Drawing for the job (mm, zero at the part's lowest x, y, z). Coordinates: 2 decimals unless noted, no trailing zeros. Order: outer loops, then holes, each group sorted by start corner. A loop starts at its lowest first (then second) coordinate and runs counter-clockwise, first axis right, second up.
1) Pin check, flat tips, straight feed: pin 1 Ø5 at (y, z) = (40, 4) entering from +X; pin 2 Ø2.5 at (x, z) = (43, 7.5) entering from -Y; pin 3 Ø3.5 at (x, z) = (12, 8.5) entering from +Y; pin 4 Ø2 at (y, z) = (71, 6) entering from +X. Stop position of each tip, or through.
2) Cut at A-A (y = 43.5). List the corners of the cut face in (x, z), and give its area (3 significant figures).
3) Wall check: L1, parallel to Y at x = 31.5, z = 12.75; L2, parallel to Y at x = 28, z = 13.5; L3, parallel to X at y = 8, z = 13.75. Give the ranges that are in metal, low to high.
4) Cut at C-C (y = 71). List the corners of the cut face in (x, z).
5) Cut at B-B (x = 34). List the corners of the cut face in (y, z).
6) Cut at D-D (z = 1). List the corners of the cut face in (x, y).
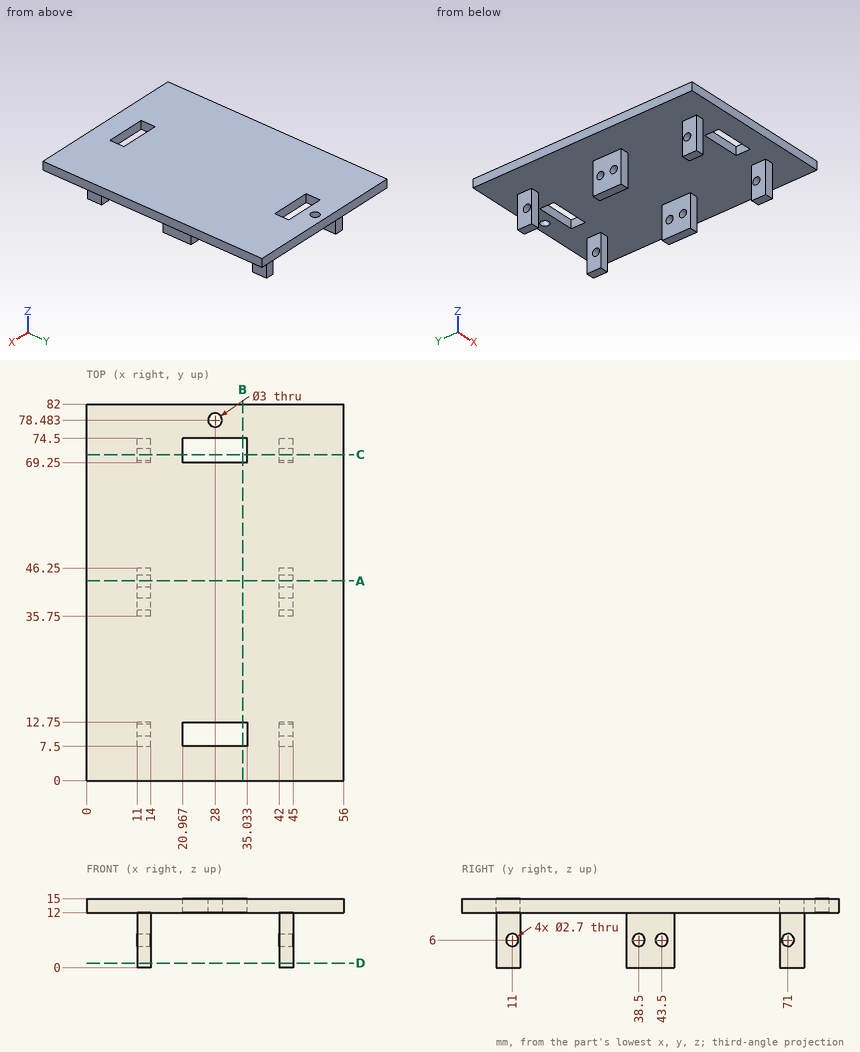
Geometry check:
1. pin 1: stops at x = 45
1. pin 2: stops at y = 7.5
1. pin 3: stops at y = 74.5
1. pin 4: passes through
2. outline: (0, 12) - (11, 12) - (11, 7.35) - (14, 7.35) - (14, 12) - (42, 12) - (42, 7.35) - (45, 7.35) - (45, 12) - (56, 12) - (56, 15) - (0, 15) - close; (11, 0) - (14, 0) - (14, 4.65) - (11, 4.65) - close; (42, 0) - (45, 0) - (45, 4.65) - (42, 4.65) - close
2. area: 224 mm2
3. L1: y = 0 to 7.5, 12.75 to 69.25, 74.5 to 82
3. L2: y = 0 to 7.5, 12.75 to 69.25, 74.5 to 76.98, 79.98 to 82
3. L3: x = 0 to 20.97, 35.03 to 56
4. outline: (0, 12) - (11, 12) - (11, 7.35) - (14, 7.35) - (14, 12) - (20.97, 12) - (20.97, 15) - (0, 15) - close; (11, 0) - (14, 0) - (14, 4.65) - (11, 4.65) - close; (35.03, 12) - (42, 12) - (42, 7.35) - (45, 7.35) - (45, 12) - (56, 12) - (56, 15) - (35.03, 15) - close; (42, 0) - (45, 0) - (45, 4.65) - (42, 4.65) - close
5. outline: (0, 12) - (7.5, 12) - (7.5, 15) - (0, 15) - close; (12.75, 12) - (69.25, 12) - (69.25, 15) - (12.75, 15) - close; (74.5, 12) - (82, 12) - (82, 15) - (74.5, 15) - close
6. outline: (11, 7.5) - (14, 7.5) - (14, 12.75) - (11, 12.75) - close; (11, 35.75) - (14, 35.75) - (14, 46.25) - (11, 46.25) - close; (11, 69.25) - (14, 69.25) - (14, 74.5) - (11, 74.5) - close; (42, 7.5) - (45, 7.5) - (45, 12.75) - (42, 12.75) - close; (42, 35.75) - (45, 35.75) - (45, 46.25) - (42, 46.25) - close; (42, 69.25) - (45, 69.25) - (45, 74.5) - (42, 74.5) - close
